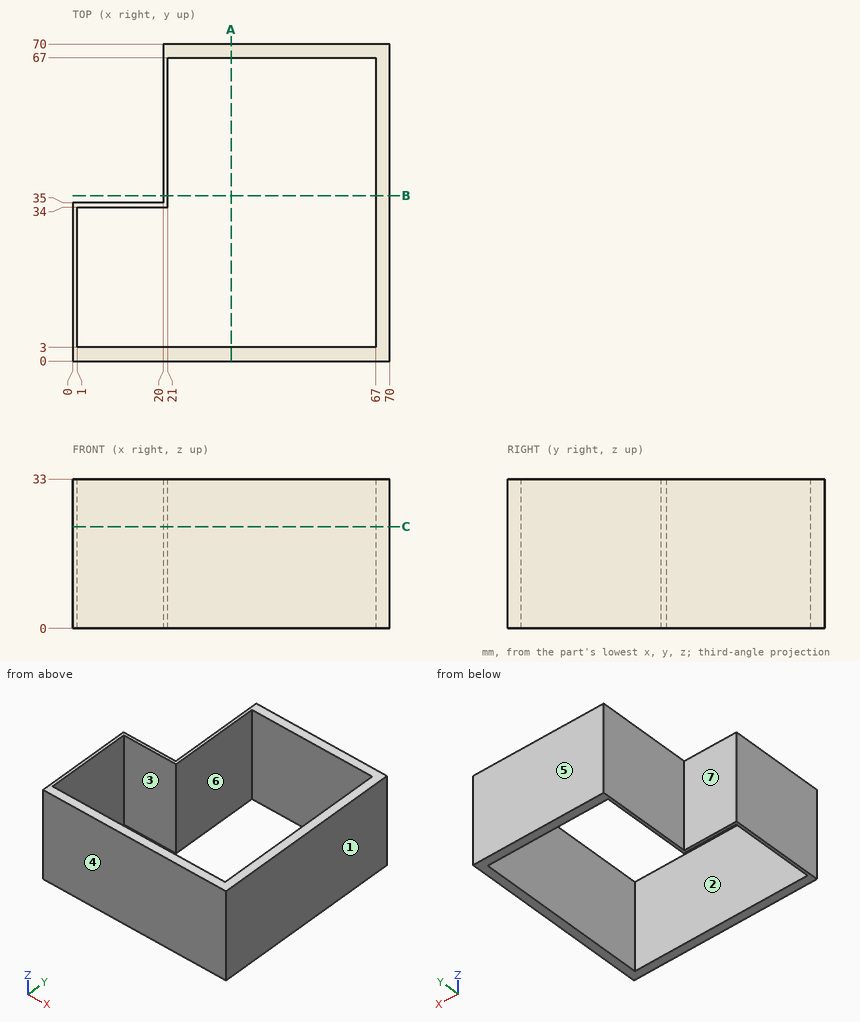
Source: three-view drawing plus pictorial views. Frame: mm from the lowest corner of the part. A direction names the side the tool comes from. Give positions to 0.01 mm unless a question says otherwise; leave off trailing zeros. Write each loop counter-clockwise with the first axis right and the second up, starting at its lowest first coordinate (ties: lowest second). Pieces come first, ordered by that corner, then holes. Notation, with made-up numbers: (55.5, -9.75) -> (89.5, -9.75) arc R16 ccw to (89.5, 7.25) -> close; hole circle Ø8 at (30, 9). An arc over 180 degrees is marked (long way). Write item = value, one per line.
Q1. First-contact query: pin 1 (1 mm diameter, centred on x = 16.5, y = 34.5, fed in from -Z); pin 2 (10 mm diameter, centred on x = 7, z = 21.5, fed in from +Y); pin 3 (10 mm diameter, centred on y = 54.5, z = 22, fed in from -X); pin 4 (12 mm diameter, centred on x = 30, y = 41.5, fed in from -Z). Flat tips, straight axial feed; report the tip coordinate or a pass-through.
Here are the results:
pin_1 = 0
pin_2 = 35
pin_3 = 20
pin_4 = through
Q2. Mould query, pull axis X, two halves, no side actions, for the marked faces 1, 2, 3 and 4. Classes: +X half, -X half, draft (parallel to the pull), parting line (faces both ways), or undercut.
Here are the results:
face_1 = +X half
face_2 = undercut
face_3 = undercut
face_4 = draft
Q3. Cut plane A-A on x = 35. Return loops of the section in (y, z).
Here are the results:
outline = (0, 0) -> (3, 0) -> (3, 33) -> (0, 33) -> close; (67, 0) -> (70, 0) -> (70, 33) -> (67, 33) -> close
Q4. Reachability of the marked faces 5, 6 and 7 from +Z, -Z, +X, -X, +Y, -Y: full face, straight path, thin tool, end or side. Return the list, or none.
Here are the results:
face_5 = +Z, -Z, +X, -X, +Y
face_6 = +Z, -Z
face_7 = +Z, -Z, -X, +Y
Q5. Line query: line 1 (X direction, y = 55, z = 30); line 2 (Y direction, x = 7, z = 29); line 3 (X direction, y = 7.5, z = 14.5). Output: solid intervals per line, ascending. Write a range as from..to.
Here are the results:
line_1 = 20..21, 67..70
line_2 = 0..3, 34..35
line_3 = 0..1, 67..70
Q6. Cut plane C-C on z = 22.5. Return loops of the section in (x, y).
Here are the results:
outline = (0, 0) -> (70, 0) -> (70, 70) -> (20, 70) -> (20, 35) -> (0, 35) -> close; hole (1, 3) -> (67, 3) -> (67, 67) -> (21, 67) -> (21, 34) -> (1, 34) -> close
Q7. Cut plane B-B on y = 36.5. Return loops of the section in (x, z), then the cut area to 3 significant figures.
Here are the results:
outline = (20, 0) -> (21, 0) -> (21, 33) -> (20, 33) -> close; (67, 0) -> (70, 0) -> (70, 33) -> (67, 33) -> close
area = 132 mm²
